Read the model definition and answer for the solid it produces. Units are mm, in the model's axes. Give positions to 0.01 mm unless a question says otherwise; leave off trailing zeros. Write each loop counter-clockwise with the first axis right and the second up, starting at its lowest first coordinate (ties: lowest second). Pieces come first, ordered by that corner, then holes.
```python
from build123d import *

# Parameters (mm, degrees)
CUT_EXTRUDE1_REACH = 18.605
SKETCH2_W          = 0.5
SKETCH2_H          = 8.115923769


with BuildPart() as part:
    # Sketch1 → Revolve1 (revolve)
    with BuildSketch(Plane(origin=(0, 0, 0), x_dir=(0, 0, -1), z_dir=(1, 0, 0)), mode=Mode.PRIVATE) as revolve1_sk:
        Polygon((0, 8.115923769), (0, 5), (12, 5), (12, 6), align=None)
    revolve(revolve1_sk.sketch.rotate(Axis((0, 0, -14.189132044), (0, 0, 1)), 90), axis=Axis((0, 0, -14.189132044), (0, 0, 1)))

    # Sketch2 → Cut-Extrude1 (cut, up to next)
    with BuildSketch(Plane.XY, mode=Mode.PRIVATE) as cut_extrude1_sk1:
        with Locations((0, 4.057961885)):
            Rectangle(SKETCH2_W, SKETCH2_H)
    cut_extrude1_tool1 = extrude(cut_extrude1_sk1.sketch, amount=-CUT_EXTRUDE1_REACH, mode=Mode.PRIVATE) & part.part
    add(cut_extrude1_tool1.solids().sort_by_distance((0, 4.057962, 0))[0], mode=Mode.SUBTRACT)


solid = part.part
```
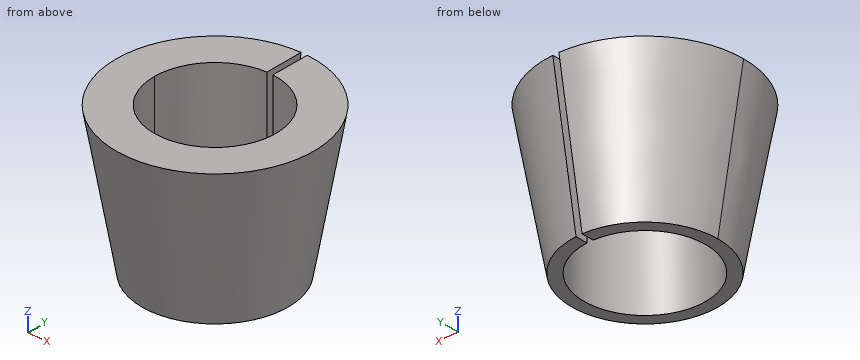
Item 1: Find the intervals of material crossed by line 1 along X through (y, z) = (5.5, -8.75); line 2 along Y through (x, z) = (-0.5, -10.75); line 3 along X through (y, z) = (5.75, -5.25), in increasing order.
Result set:
line 1: x = -3.6 to -0.25, 0.25 to 3.6
line 2: y = -6.2 to -4.97, 4.97 to 6.2
line 3: x = -4.32 to -0.25, 0.25 to 4.32
Item 2: Section A-A (x = 0) is taken. Write down the section's boundary in (y, z), and give its area (3 significant figures).
Result set:
outline: (-8.12, 0) - (-6, -12) - (-5, -12) - (-5, 0) - close
area: 24.7 mm2
Item 3: Each of these flat-tipped pins is pushed along its axis until it touches: pin 1 Ø2.5 at (y, z) = (6, -4.5) entering from +X; pin 2 Ø6 at (y, z) = (-5.5, -3) entering from +X; pin 3 Ø9 at (x, y) = (0, 0) entering from -Z; pin 4 Ø3 at (x, z) = (5, -9.5) entering from +Y. Where does it stop, or does it pass through?
Result set:
pin 1: stops at x = 5.61
pin 2: stops at x = 7.3
pin 3: passes through
pin 4: stops at y = 5.46
Item 4: Section B-B (z = -3) is taken. Write down the section's boundary in (x, y).
Result set:
outline: (-0.25, 4.99) - (-0.25, 7.58) arc R7.59 ccw (long way) to (0.25, 7.58) - (0.25, 4.99) arc R5 cw (long way) to start
